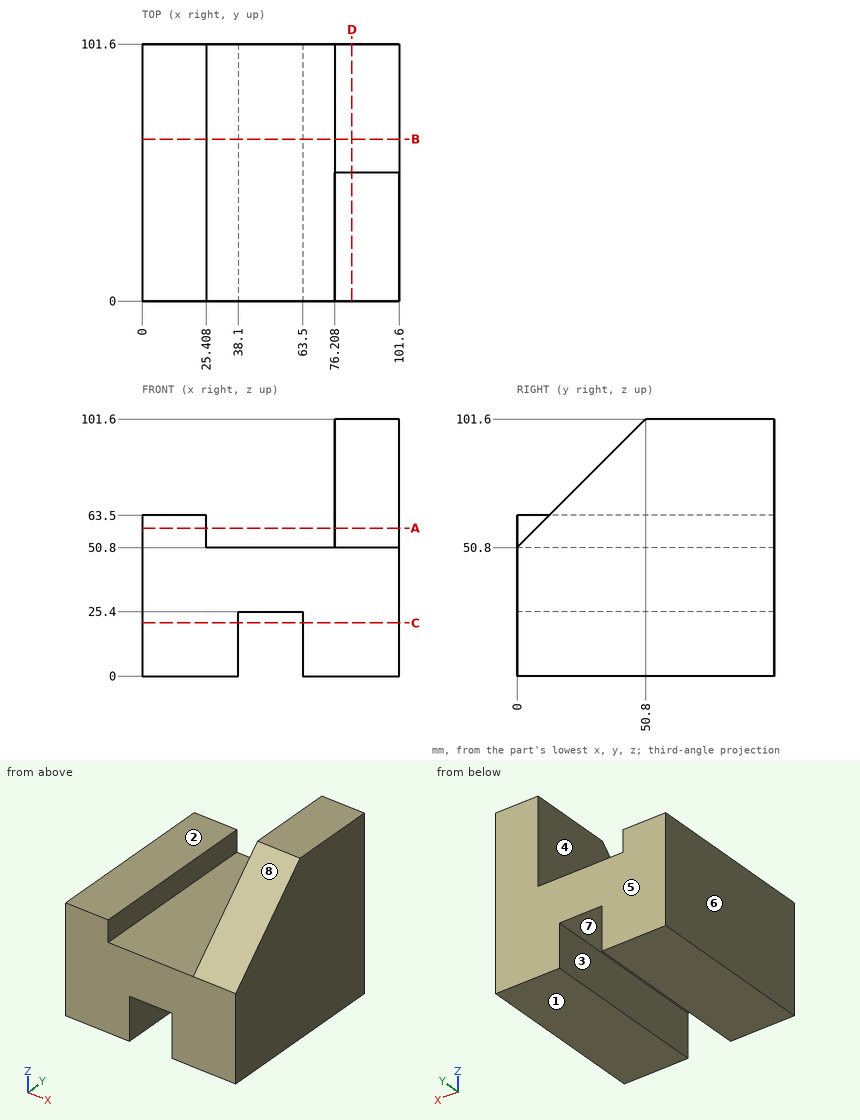
Verification items for this drawing (mm, ordinates from the low corner). A direction names the side the tool comes from. Coordinates: 2 decimals unless noted, no trailing zeros. Write each loop counter-clockwise with the first axis right and the second up, starting at its lowest first coordinate (ties: lowest second). Pieces come first, ordered by that corner, then holes. Notation, with made-up numbers: (37.25, -9) -> (85.25, -9) arc R22 cw to (85.25, 7) -> close; hole circle Ø3 at (52.25, 25.5). An arc over 180 degrees is marked (long way). Use CSV: the item, a comma, the result in double quotes. Start each with the question number.
Item 1: Cross-section at D-D, the plane x = 83. Record the cut outline in (y, z).
Item 2: Cross-section at C-C, the plane z = 21. Record the cut outline in (x, y).
Item 3: Thickness scan on line 1 (X direction, y = 45, z = 19); line 2 (X direction, y = 15, z = 58); line 3 (Z direction, x = 27, y = 55.5). Record the ranges inside material, lowest first.
Item 4: Mould release check, pull along X, two halves, no side actions. Record for the marked faces 6, 7 and 8: released by +X, released by -X, zero draft, split by the parting line, or undercut.
Item 5: Cross-section at A-A, the plane z = 58.5. Record the cut outline in (x, y), plus the area to 3 significant figures.
Item 6: Cross-section at B-B, the plane y = 64. Record the cut outline in (x, z), plus the area to 3 significant figures.
Item 7: Set-up check for the marked faces 1, 2, 3, 4 and 5: record each of +Z, -Z, +X, -X, +Y, -Y from which the full face is reachable in a straight line by a thin tool's end or side.
Item 8: Depth check by flat-ended pin: pin 1 Ø7.5 at (x, y) = (54, 68.5) entering from -Z; pin 2 Ø8 at (y, z) = (83.5, 68) entering from -X; pin 3 Ø7.5 at (x, y) = (17.5, 37.5) entering from +Z. Enter the tip coordinate at first touch or a pass-through.
Answers:
1,outline,"(0, 0) -> (101.6, 0) -> (101.6, 101.6) -> (50.8, 101.6) -> (0, 50.8) -> close"
2,outline,"(0, 0) -> (38.1, 0) -> (38.1, 101.6) -> (0, 101.6) -> close; (63.5, 0) -> (101.6, 0) -> (101.6, 101.6) -> (63.5, 101.6) -> close"
3,line 1,"0 to 38.1, 63.5 to 101.6"
3,line 2,"0 to 25.41, 76.21 to 101.6"
3,line 3,"0 to 50.8"
4,face 6,"released by -X"
4,face 7,"undercut"
4,face 8,"zero draft"
5,outline,"(0, 0) -> (25.41, 0) -> (25.41, 101.6) -> (0, 101.6) -> close; (76.21, 7.7) -> (101.6, 7.7) -> (101.6, 101.6) -> (76.21, 101.6) -> close"
5,area,"4,970 mm^2"
6,outline,"(0, 0) -> (38.1, 0) -> (38.1, 25.4) -> (63.5, 25.4) -> (63.5, 0) -> (101.6, 0) -> (101.6, 101.6) -> (76.21, 101.6) -> (76.21, 50.8) -> (25.41, 50.8) -> (25.41, 63.5) -> (0, 63.5) -> close"
6,area,"6,130 mm^2"
7,face 1,"-Z, +X, -X, +Y, -Y"
7,face 2,"+Z, -X, +Y, -Y"
7,face 3,"-Z, +Y, -Y"
7,face 4,"+Z, +Y, -Y"
7,face 5,"+Z, -Z, +X, -X, +Y"
8,pin 1,"z = 25.4"
8,pin 2,"x = 76.21"
8,pin 3,"z = 63.5"
